Input: part model. Units: mm. Frame: model coordinates. Coordinates: 2 decimals unless noted, no trailing zeros. Order: outer loops, then holes, each group sorted by start corner. A loop starts at its lowest first (then second) coordinate and runs counter-clockwise, first axis right, second up. Notation, with made-up numbers: (22, 41) - (48, 41) arc R27 ccw to (48, 71) - close; hole circle Ø2 at (-29, 32). An arc over 180 degrees is marked (long way). One line per question, with ' | ' between items. Start each with the question number.
Autodesk Inventor part; units mm, degrees
ref_plane "YZ Plane" through (0, 0, 0) normal (1, 0, 0) x (0, 1, 0)
ref_plane "XZ Plane" through (0, 0, 0) normal (0, 1, 0) x (-1, 0, 0)
ref_plane "XY Plane" through (0, 0, 0) normal (0, 0, 1) x (1, 0, 0)
sketch "Sketch1" plane through (0, 0, 0) normal (0, 1, 0) x (-1, 0, 0)
  line L0 (-132.5, 287.3805) -> (-122.5, 287.3805)
  line L1 (-132.5, 20) -> (-132.5, 287.3805)
  line L2 (-122.5, 20) -> (-122.5, 287.3805)
  line L3 (77.5, 287.3805) -> (87.5, 287.3805)
  line L4 (77.5, 20) -> (77.5, 287.3805)
  line L5 (87.5, 20) -> (87.5, 287.3805)
  line L6 (82.5, 0) -> (127.5, 0) construction
  line L7 (-132.5, 20) -> (-132.5, 287.3805)
  line L8 (82.5, 45) -> (-127.5, 45)
  line L9 (82.5, 155) -> (-127.5, 155)
  circle A0 centre (-127.5, 265) radius 1.6
  circle A1 centre (-127.5, 155) radius 1.6
  circle A2 centre (-127.5, 45) radius 1.6
  circle A3 centre (82.5, 45) radius 1.6
  circle A4 centre (82.5, 155) radius 1.6
  circle A5 centre (82.5, 265) radius 1.6
  line L10 (-132.5, 287.3805) -> (87.5, 287.3805)
  line L11 (87.5, 287.3805) -> (87.5, 0)
  line L12 (87.5, 0) -> (-132.5, 0)
  line L13 (-132.5, 0) -> (-132.5, 287.3805)
  line L14 (87.5, 0) -> (-132.5, 0)
  line L15 (-132.5, 0) -> (-132.5, -22.8)
  line L16 (-132.5, -22.8) -> (87.5, -22.8)
  line L17 (87.5, -22.8) -> (87.5, 0)
  arc A6 (6, 100) -> (0, 94) centre (6, 94) ccw
  line L18 (0, 0) -> (0, 94)
  line L19 (0, 0) -> (90, 0)
  line L20 (90, 0) -> (90, 94)
  arc A7 (90, 94) -> (84, 100) centre (84, 94) ccw
  line L21 (6, 100) -> (84, 100)
  circle A8 centre (45, 47.3805) radius 11
  circle A9 centre (76.75, 79.1305) radius 5.75
  circle A10 centre (13.25, 15.6305) radius 5.75
  circle A11 centre (76.75, 15.6305) radius 5.75
  circle A12 centre (13.25, 79.1305) radius 5.75
  circle A13 centre (117.5, 135) radius 1.8
  line L22 (112.5, 267.3805) -> (122.5, 267.3805)
  line L23 (112.5, 0) -> (112.5, 267.3805)
  line L24 (112.5, 0) -> (122.5, 0)
  line L25 (122.5, 0) -> (122.5, 267.3805)
  circle A14 centre (117.5, 25) radius 1.8
  circle A15 centre (117.5, 245) radius 1.8
  circle A16 centre (-92.5, 135) radius 1.8
  line L26 (-97.5, 267.3805) -> (-87.5, 267.3805)
  line L27 (-97.5, 0) -> (-97.5, 267.3805)
  line L28 (-97.5, 0) -> (-87.5, 0)
  line L29 (-87.5, 0) -> (-87.5, 267.3805)
  circle A17 centre (-92.5, 245) radius 1.8
  circle A18 centre (-92.5, 25) radius 1.8
  point P0 (-62.5, 0)
  point P1 (52.5, -20)
  dimension "d0" = 45
  dimension "d2" = 110
  dimension "d4" = 3.2
  dimension "d5" = 3.2
  dimension "d6" = 3.2
  dimension "d7" = 3.2
  dimension "d8" = 3.2
  dimension "d9" = 3.2
  dimension "d12" = 22.8
extrude "Extrusion1" add sketch "Sketch1" along normal blind 3 contours L0 L2 L8 L27 L12 L13 L1 | L10 L4 L9 L29 L26 L27 L2 | L9 L27 L8 L2 | L3 L5 A7 L21 L4 | L27 L26 L29 L9 | L9 L29 L8 L27 | L4 L21 A6 L18 L8 L29 L9 | L27 L8 L29 L12 | L5 L11 L12 L18 L8 A8 L4 A9 L21 A7 | L4 A9 L8 A8 L18 A6 L21 | L29 L8 L18 L12 | A9 L4 | L4 A9 | A8 L8 | L8 A8 | A10 | A11 | A12 | A16 | A17 | A18
fillet "Fillet1" radius 20 2 edges at (132.5, 1.5, 0) (-87.5, 1.5, 0)
sketch "Sketch3" plane through (0, 0, 0) normal (0, -1, 0) x (1, 0, 0)
  line L0 (92.3, 110.2305) -> (17.7, 110.2305)
  circle A0 centre (23.25, 99.1305) radius 4.9999
  circle A1 centre (86.75, 99.1305) radius 4.9999
  circle A2 centre (23.25, 35.6305) radius 4.9999
  circle A3 centre (86.75, 35.6305) radius 4.9999
  line L1 (10, 20) -> (10, 114)
  line L2 (100, 20) -> (100, 114)
  line L3 (112.5, 0) -> (-67.5, 0)
  line L4 (132.5, 287.3805) -> (132.5, 20)
  line L5 (-87.5, 20) -> (-87.5, 287.3805)
  line L6 (-87.5, 287.3805) -> (132.5, 287.3805)
  arc A4 (-87.5, 20) -> (-67.5, 0) centre (-67.5, 20) ccw
  line L7 (112.5, 0) -> (-67.5, 0)
  arc A5 (112.5, 0) -> (132.5, 20) centre (112.5, 20) ccw
  line L8 (132.5, 287.3805) -> (132.5, 20)
  line L9 (-87.5, 287.3805) -> (132.5, 287.3805)
  line L10 (-87.5, 20) -> (-87.5, 287.3805)
  circle A6 centre (127.5, 155) radius 1.6
  circle A7 centre (127.5, 45) radius 1.6
  circle A8 centre (-82.5, 45) radius 1.6
  circle A9 centre (-82.5, 155) radius 1.6
  circle A10 centre (127.5, 265) radius 1.6
  circle A11 centre (-82.5, 265) radius 1.6
  circle A12 centre (86.75, 99.1305) radius 10
  circle A13 centre (86.75, 35.6305) radius 10
  circle A14 centre (23.25, 99.1305) radius 10
  circle A15 centre (23.25, 35.6305) radius 10
  point P0 (0, 0)
  dimension "d18" = 20
  dimension "d19" = 20
  dimension "d20" = 20
  dimension "d21" = 20
extrude "Extrusion2" cut sketch "Sketch3" against normal up to surface (3 mm away) contours A0 | A1 | A2 | A3 | A12 | A13 | A14 | A15
equation "\"BendRadius\" = Thickness"
equation "\"BendReliefWidth\" = Thickness"
equation "\"BendReliefDepth\" = 0.5 * Thickness"
equation "\"CornerReliefSize\" = 4 * Thickness"
equation "\"MinimumRemnant\" = 2 * Thickness"
equation "\"TransitionRadius\" = BendRadius"
equation "\"JacobiRadiusSize\" = Thickness"
equation "\"GapSize\" = Thickness"
properties part number "obudowa_zewnetrzna_przod" material "ABS Plastic"
(1) Section A-A (x = 23.25). Output: boundary loops of the cut face in (y, z).
(2) Section B-B (y = 0.95). State how many separate pieces and enclosed holes the cut face has, then the cut area to 3 significant figures.
(3) Draft query along X for faces 1 (the face through (-81.486, 1.521, 5.703)), 2 (the face through (126.797, 1.521, 6.014)), 3 (the face through (78.81, 1.48, 93.05)), 4 (the face through (24, 0, 146)). Return one class per face: +X half, -X half, draft (parallel to the pull), parting line (faces both ways), or undercut.
(4) Material intervals for line 1 along X through (y, z) = (1.6, 155); line 2 along X through (y, z) = (1.7, 102); line 3 along Z through (x, y) = (-71.5, 2.55), sorted ascending. Write a range as from..to.
(5) Pin query (flat end, axial travel): pin 1 (3 mm diameter, centred on x = -16, z = 257.5, fed in from -Y); pin 2 (18 mm diameter, centred on x = 23.25, z = 99.13, fed in from +Y). Return the tip coordinate at first contact, or that it passes through.
Worked answers:
1) outline: (0, 0) - (3, 0) - (3, 25.63) - (0, 25.63) - close; (0, 45.63) - (3, 45.63) - (3, 89.13) - (0, 89.13) - close; (0, 109.13) - (3, 109.13) - (3, 287.38) - (0, 287.38) - close
2) separate pieces: 1 | enclosed holes: 10 | area: 61,700 mm²
3) face 1: -X half | face 2: +X half | face 3: undercut | face 4: draft
4) line 1: x = -87.5..-84.1, -80.9..125.9, 129.1..132.5 | line 2: x = -87.5..13.67, 32.83..77.17, 96.33..132.5 | line 3: z = 0.4..287.38
5) pin 1: stops at y = 0 | pin 2: passes through
